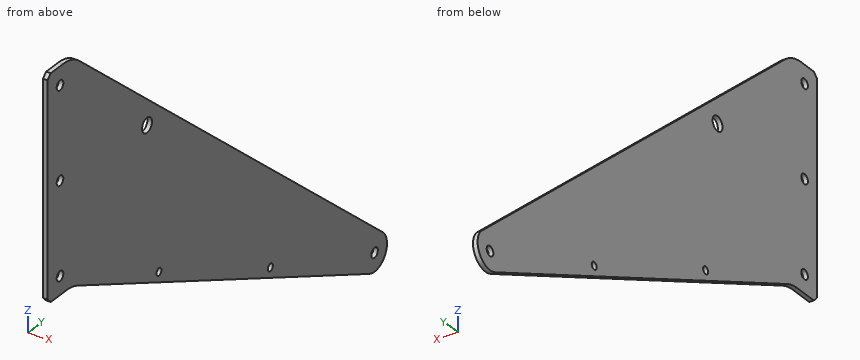
```python
from build123d import *

# Parameters (mm, degrees)
SKETCH2_R           = 5.0419
SKETCH2_R_2         = 3.3782
BOSS_EXTRUDE2_DEPTH = 3.175
SKETCH3_R           = 3.3782
SKETCH3_R_2         = 2.54
CUT_EXTRUDE1_DEPTH  = 4.175
CHAMFER1_SIZE       = 3.175
FILLET1_R           = 25.4


with BuildPart() as part:
    # Sketch2 → Boss-Extrude2 (new body)
    with BuildSketch(Plane(origin=(0, 0, 0), x_dir=(0, 0, -1), z_dir=(1, 0, 0))):
        with BuildLine():
            Line((0, 0), (0, 25.4))
            Line((0, 25.4), (270.911778308, 342.321467673))
            ThreePointArc((270.911778308, 342.321467673), (287.412585426, 344.765407005), (292.10095893, 328.757014554))
            Line((292.10095893, 328.757014554), (152.4, 25.4))
            Line((152.4, 25.4), (152.4, 0))
            Line((152.4, 0), (0, 0))
        make_face()
        with Locations((82.55, 101.6)):
            Circle(SKETCH2_R, mode=Mode.SUBTRACT)
        with Locations((280.565394007, 334.069334376)):
            Circle(SKETCH2_R_2, mode=Mode.SUBTRACT)
    extrude(amount=BOSS_EXTRUDE2_DEPTH)

    # Sketch3 → Cut-Extrude1 (cut, through all)
    with BuildSketch(Plane(origin=(3.175, 0, 0), x_dir=(0, 0, -1), z_dir=(1, 0, 0))):
        with Locations((12.7, 12.7)):
            Circle(SKETCH3_R)
        with Locations((76.2, 12.7)):
            Circle(SKETCH3_R)
        with Locations((139.7, 12.7)):
            Circle(SKETCH3_R)
        with Locations((238.526483092, 227.602177824)):
            Circle(SKETCH3_R_2)
        with Locations((186.119185797, 113.801088912)):
            Circle(SKETCH3_R_2)
    extrude(amount=-CUT_EXTRUDE1_DEPTH, mode=Mode.SUBTRACT)

    # Chamfer1
    chamfer1_edges = [part.edges().sort_by_distance(p)[0] for p in [
        (1.5875, 0, 0),
        (1.5875, 0, -152.4),
    ]]
    chamfer(chamfer1_edges, length=CHAMFER1_SIZE)

    # Fillet1
    fillet1_edges = [part.edges().sort_by_distance(p)[0] for p in [
        (1.5875, 25.4, 0),
        (1.5875, 25.4, -152.4),
    ]]
    fillet(fillet1_edges, radius=FILLET1_R)


solid = part.part
```
The model under review builds one solid part; all positions refer to its coordinate system, in mm. Round coordinates to 2 decimals unless told otherwise and drop trailing zeros. Loops run counter-clockwise (first coordinate to the right, second up) from the corner with the lowest first, then second, coordinate; pieces in that order, holes last. Notation, with made-up numbers: (64, -35) - (70, -35) arc R15 ccw to (70, -25) - close; hole circle Ø4 at (61.5, -22). An arc over 180 degrees is marked (long way). Write each question's results on one line, items separated by ' | '. Start each with the question number.
Q1. Insertion check: P1, Ø3, axis at y = 227.6, z = -238.53, coming from the +X side; P2, Ø8, axis at y = 12.7, z = -139.7, coming from the -X side; P3, Ø1, axis at x = 2, y = 123, coming from the +Z side; P4, Ø1.6, axis at x = 2, y = 13, coming from the -Z side. Each pin has a flat end and moves straight along its axis. Give the tip position at first contact, or say it passes through.
Q2. Take a section at C-C on z = -60.5. Give the boundary of the cut face in (x, y) (3 decimals).
Q3. Take a section at D-D on y = 238. Give the boundary of the cut face in (x, z) (3 decimals), plus the area to 3 significant figures.
Q4. Take a section at B-B on y = 101.6. Give the boundary of the cut face in (x, z) (3 decimals), plus the area to 3 significant figures.
Q5. Wall thickness on line 1 along Y through (x, z) = (0.8, -82.55); line 2 along Z through (x, y) = (2.1, 121.5); line 3 along Y through (x, z) = (0.7, -190): over which ranges is each line inside the solid? List them lowest first. Write a range as [from, to].
Q6. Take a section at A-A on x = 0.8. Give the boundary of the cut face in (y, z) (3 decimals).
Data:
1) P1: passes through | P2: stops at x = 0 | P3: stops at z = -83 | P4: stops at z = -152.4
2) outline: (0, 0) - (3.175, 0) - (3.175, 96.175) - (0, 96.175) - close
3) outline: (0, -250.306) - (3.175, -250.306) - (3.175, -181.735) - (0, -181.735) - close | area: 218 mm²
4) outline: (0, -187.491) - (3.175, -187.491) - (3.175, -87.592) - (0, -87.592) - close; (0, -77.508) - (3.175, -77.508) - (3.175, -65.138) - (0, -65.138) - close | area: 356 mm²
5) line 1: y = [0, 96.56], [106.64, 121.97] | line 2: z = [-196.66, -82.15] | line 3: y = [107.05, 247.67]
6) outline: (0, -149.225) - (3.175, -152.4) - (19.832, -152.4) arc R25.4 cw to (30.457, -154.729) - (328.757, -292.101) arc R12.7 ccw to (342.321, -270.912) - (32.528, -6.093) arc R25.4 ccw to (16.023, 0) - (3.175, 0) - (0, -3.175) - close; hole circle Ø6.756 at (12.7, -139.7); hole circle Ø6.756 at (12.7, -76.2); hole circle Ø6.756 at (12.7, -12.7); hole circle Ø10.084 at (101.6, -82.55); hole circle Ø5.08 at (113.801, -186.119); hole circle Ø5.08 at (227.602, -238.526); hole circle Ø6.756 at (334.069, -280.565)
